Autodesk Inventor part; units mm, degrees
ref_plane "작업 평면1" through (-15, 23, -25) normal (-1, 0, 0) x (0, 0, 1)
ref_plane "YZ Plane" through (0, 0, 0) normal (1, 0, 0) x (0, 1, 0)
ref_plane "XZ Plane" through (0, 0, 0) normal (0, 1, 0) x (-1, 0, 0)
sketch "스케치1" plane through (0, 0, 0) normal (0, 0, 1) x (1, 0, 0)
  line L0 (-5, -33) -> (5, -33)
  line L1 (5, -33) -> (5, 33)
  line L2 (5, 33) -> (-5, 33)
  line L3 (-5, 33) -> (-5, -33)
  line L4 (-5, -33) -> (5, 33) construction
  line L5 (5, -33) -> (-5, 33) construction
  line L6 (-5, 33) -> (-35, 33)
  line L7 (-35, 33) -> (-35, 23)
  line L8 (-35, 23) -> (-5, 23)
  line L9 (-5, 23) -> (-5, 33)
  line L10 (0, 0) -> (-11.0402, 0)
  line L11 (-5, -33) -> (-35, -33)
  line L12 (-35, -33) -> (-35, -23)
  line L13 (-35, -23) -> (-5, -23)
  point P0 (-5, 23)
  point P1 (-5, -23)
  dimension "d0" = 66
  dimension "d1" = 10
  dimension "d2" = 10
  dimension "d3" = 30
extrude "돌출1" add sketch "스케치1" along normal mid plane 50
sketch "스케치2" plane through (0, 0, 25) normal (0, 0, 1) x (1, 0, 0)
  circle A0 centre (-15, 183) radius 14
  line L0 (-35, 33) -> (-35, 23)
  line L1 (-35, 33) -> (-28.9889, 183.5585)
  line L2 (5, 33) -> (-35, 33)
  line L3 (-15, 33) -> (-15, 183) construction
  line L4 (5, 33) -> (-1.0111, 183.5585)
  point P0 (0, 0)
  dimension "d6" = 28
  dimension "d17" = 6
  dimension "d7" = 150
extrude "돌출2" add sketch "스케치2" against normal blind 10
ref_plane "작업 평면1" through (-15, 23, -25) normal (-1, 0, 0) x (0, 0, 1)
sketch "스케치3" plane through (-15, 23, -25) normal (-1, 0, 0) x (0, 0, 1)
  line L0 (40, 160.5585) -> (40, 10)
  line L1 (0, 10) -> (40, 10)
  line L2 (40, 144.5585) -> (0, 10)
  line L3 (45.7513, 142.8488) -> (8.0431, 16)
  line L4 (8.0431, 16) -> (34, 16)
  line L5 (34, 16) -> (34, 160.5585)
  line L6 (34, 16) -> (20, 56.2226)
  line L7 (34, 34.2526) -> (22.9265, 66.0672)
  point P0 (25, -23)
  point P1 (34, 103.318)
  point P2 (34, 124.3747)
  point P3 (40, 123.5018)
  dimension "d10" = 16
  dimension "d11" = 6
  dimension "d12" = 6
extrude "돌출3" add sketch "스케치3" along normal mid plane 10 contours L0 L3 L5 L2 | L0 L1 L2 L5 L3 | L7 L5 L6 L3
sketch "스케치4" plane through (0, 0, 25) normal (0, 0, 1) x (1, 0, 0)
  line L0 (-35, 33) -> (-28.9889, 183.5585)
  line L1 (5, 33) -> (-1.0111, 183.5585)
  line L2 (-35, 33) -> (5, 33)
  arc A0 (-1.0111, 183.5585) -> (-28.9889, 183.5585) centre (-15, 183) ccw
  line L3 (-7.0064, 183.3192) -> (-1.2443, 39)
  line L4 (-1.2443, 39) -> (-28.7557, 39)
  line L5 (-28.7557, 39) -> (-22.9936, 183.3192)
  arc A1 (-7.0064, 183.3192) -> (-22.9936, 183.3192) centre (-15, 183) ccw
  line L6 (-1.2443, 39) -> (-27.6994, 65.4551)
  line L7 (-1.5972, 47.8382) -> (-27.3737, 73.6146)
  line L8 (-27.3737, 73.6146) -> (-3.5765, 97.4118)
  line L9 (-3.9022, 105.5713) -> (-27.0208, 82.4528)
  line L10 (-3.9022, 105.5713) -> (-25.2456, 126.9147)
  line L11 (-25.2456, 126.9147) -> (-5.5411, 146.6192)
  line L12 (-5.5411, 146.6192) -> (-23.7326, 164.8107)
  line L13 (-23.7326, 164.8107) -> (-6.2674, 164.8107)
  line L14 (-21.003, 131.1573) -> (-4.2551, 114.4095)
  line L15 (-15.2473, 164.8107) -> (-5.894, 155.4574)
  line L16 (-24.8927, 135.7528) -> (-9.7837, 150.8618)
  point P0 (0, 0)
  point P1 (-5.2153, 138.4597)
  dimension "d15" = 6
  dimension "d16" = 45
  dimension "d17" = 6
  dimension "d18" = 90
  dimension "d19" = 6
  dimension "d23" = 6
extrude "돌출4" cut sketch "스케치4" against normal blind 10 contours L3 L15 L13 | L12 L16 L5 | L3 L14 L11 | L10 L9 L5 | L3 L7 L8 | L6 L4 L5
properties part number "전체 형상"
Check sheet for the modelled part. Datum: model origin and axes. Units: mm. A direction names the side the tool comes from. Give positions to 0.01 mm unless a question says otherwise; leave off trailing zeros. Order: outer loops, then holes, each group sorted by start corner. A loop starts at its lowest first (then second) coordinate and runs counter-clockwise, first axis right, second up. Notation, with made-up numbers: (1.5, 54.25) - (13.5, 54.25) arc R21 ccw to (13.5, 77.25) - close; hole circle Ø1 at (-6.75, 73). An arc over 180 degrees is marked (long way). Answer as CSV lines item,"result".
1. Scan lines: probe 1 along Y at (x, z) = (-21.5, -10.5); probe 2 along X at (y, z) = (7, -7.5); probe 3 along Z at (x, y) = (-17.5, 60). Record each from-to range of solid material in increasing order. Write a range as from..to.
Result sheet:
probe 1,"-33..-23, 23..33"
probe 2,"-5..5"
probe 3,"-16.97..-10.71, 1.69..8.04, 9..25"
2. Section check C-C (z = -11.5). Record the boundary of the cut face in (x, y).
Result sheet:
outline,"(-35, -33) - (5, -33) - (5, 33) - (-10, 33) - (-10, 39) - (-20, 39) - (-20, 33) - (-35, 33) - (-35, 23) - (-5, 23) - (-5, -23) - (-35, -23) - close; (-20, 57.36) - (-10, 57.36) - (-10, 78.41) - (-20, 78.41) - close"
3. Tool access check on faces 5 (the face through (-6.4, 116.1, 15)), 6 (the face through (-4.907, 130.74, 20.07)), 7 (the face through (5, 0, 0)), 8 (the face through (-16, 106, 15)), 9 (the face through (-15, -33, 0)). Record the directions out of +Z, -Z, +X, -X, +Y, -Y that give a thin tool (end or side, any length) a straight path to the whole face; none if there is none.
Result sheet:
face 5,"-Z, +Y"
face 6,"+Z, -Z"
face 7,"+Z, -Z, +X, +Y, -Y"
face 8,"+Z"
face 9,"+Z, -Z, +X, -X, -Y"
4. Section check B-B (y = 86.5). Record the boundary of the cut face in (x, z).
Result sheet:
outline,"(-32.86, 15) - (-26.86, 15) - (-26.86, 25) - (-32.86, 25) - close; (-22.97, 15) - (-20, 15) - (-20, 9) - (-10, 9) - (-10, 15) - (-14.49, 15) - (-14.49, 25) - (-22.97, 25) - close; (-20, -9.1) - (-10, -9.1) - (-10, -1.18) - (-20, -1.18) - close; (-3.14, 15) - (2.86, 15) - (2.86, 25) - (-3.14, 25) - close"
5. Section check D-D (z = -21). Record the boundary of the cut face in (x, y), then the cut area to 3 significant figures.
Result sheet:
outline,"(-35, -33) - (5, -33) - (5, 33) - (-10, 33) - (-10, 46.46) - (-20, 46.46) - (-20, 33) - (-35, 33) - (-35, 23) - (-5, 23) - (-5, -23) - (-35, -23) - close"
area,"1,390 mm²"
6. Section check A-A (z = 20.5). Record the boundary of the cut face in (x, y).
Result sheet:
outline,"(-35, -33) - (5, -33) - (5, 33) - (-1.01, 183.56) arc R14 ccw to (-28.99, 183.56) - (-35, 33) - (-35, 23) - (-5, 23) - (-5, -23) - (-35, -23) - close; hole (-28.76, 39) - (-1.24, 39) - (-27.7, 65.46) - close; hole (-27.37, 73.61) - (-1.6, 47.84) - (-3.58, 97.41) - close; hole (-27.02, 82.45) - (-3.9, 105.57) - (-25.25, 126.91) - close; hole (-24.89, 135.75) - (-9.78, 150.86) - (-23.73, 164.81) - close; hole (-21, 131.16) - (-4.26, 114.41) - (-5.54, 146.62) - close; hole (-15.25, 164.81) - (-5.89, 155.46) - (-6.27, 164.81) - close"
7. Go/stop test with flat-tipped pins: P1, Ø5, axis at x = -15.5, y = 98.5, coming from the +Z side; P2, Ø1, axis at x = -9.5, z = 15.5, coming from the +Y side; P3, Ø20, axis at y = 124.5, z = -2.5, coming from the -X side. Record where each tip stops, or that it passes through.
Result sheet:
P1,"z = 15"
P2,"y = 196.08"
P3,"x = -20"
8. Mould release check, pull along X, two halves, no side actions. Record for faces 1 (the face through (-6.083, 160.2, 20.07)), 2 (the face through (-5, 0, 0)), 3 (the face through (-16, 46, 15)), 4 (the face through (-27, 33, -5)): released by +X, released by -X, zero draft, split by the parting line, or undercut.
Result sheet:
face 1,"undercut"
face 2,"released by -X"
face 3,"undercut"
face 4,"zero draft"
